Print and shaded views of the part. All mm, measured from the part's lowest x, y and z. Give positions to 0.01 mm unless a question says otherwise; leave off trailing zeros. Order: outer loops, then holes, each group sorted by start corner. A loop starts at its lowest first (then second) coordinate and runs counter-clockwise, first axis right, second up. Notation, with made-up numbers: (64.25, -5) - (90.25, -5) arc R20 cw to (90.25, 17) - close; hole circle Ø2 at (-37.5, -22.5). An arc over 180 degrees is marked (long way). Answer in a Markdown table with one row per item.
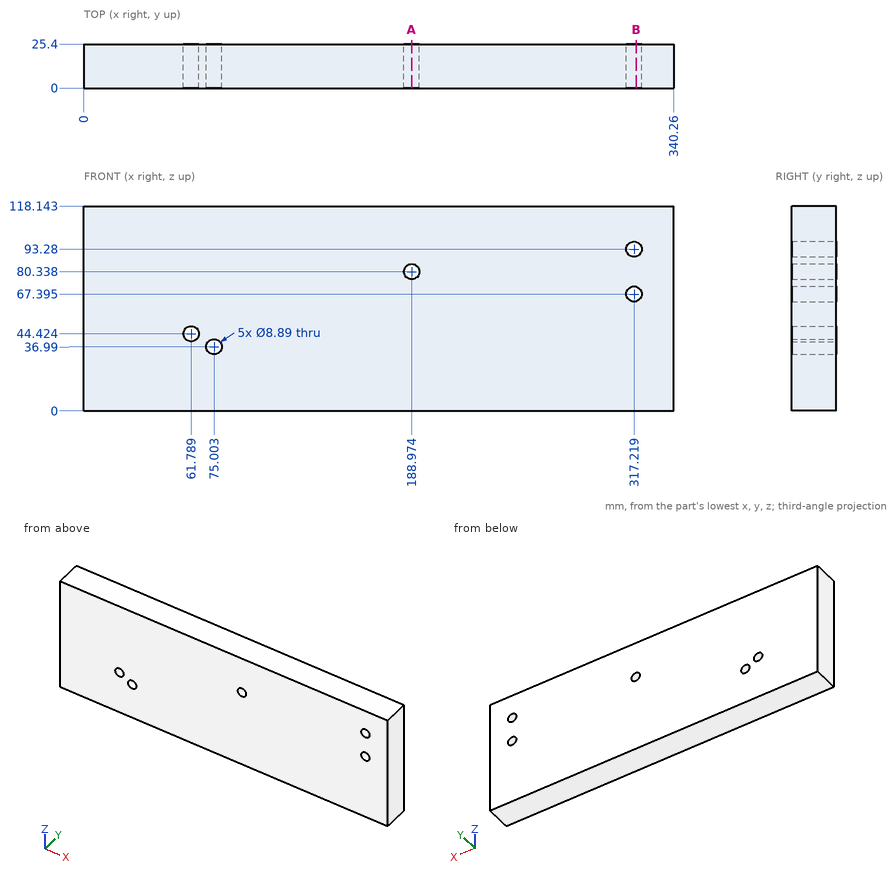
1. Cut at B-B on x = 318.5. Write the cut outline in (y, z), and give its area (3 significant figures).
Check result:
| item | result |
|---|---|
| outline | (0, 0) - (25.4, 0) - (25.4, 63.14) - (0, 63.14) - close; (0, 71.65) - (25.4, 71.65) - (25.4, 89.02) - (0, 89.02) - close; (0, 97.54) - (25.4, 97.54) - (25.4, 118.14) - (0, 118.14) - close |
| area | 2,570 mm² |
2. Probe line 1 (Z direction, x = 320, y = 16); line 2 (X direction, y = 24.25, z = 78.5); line 3 (Z direction, x = 74, y = 8.5). List the from-to ranges inside material, lowest first.
Check result:
| item | result |
|---|---|
| line 1 | z = 0 to 63.93, 70.86 to 89.81, 96.75 to 118.14 |
| line 2 | x = 0 to 184.93, 193.02 to 340.26 |
| line 3 | z = 0 to 32.66, 41.32 to 118.14 |
3. Cut at A-A on x = 189. Write the cut outline in (y, z), and give its area (4 significant figures).
Check result:
| item | result |
|---|---|
| outline | (0, 0) - (25.4, 0) - (25.4, 75.89) - (0, 75.89) - close; (0, 84.78) - (25.4, 84.78) - (25.4, 118.14) - (0, 118.14) - close |
| area | 2,775 mm² |
